from build123d import *

# Parameters (mm, degrees)
SKETCH1_W                = 39.6
SKETCH1_H                = 30
BOSS_EXTRUDE1_DEPTH      = 5
BOSS_EXTRUDE2_DEPTH      = 5.25
BOSS_EXTRUDE2_DEPTH_BACK = 4.75
BOSS_EXTRUDE3_DEPTH      = 5.25
BOSS_EXTRUDE3_DEPTH_BACK = 4.75
SKETCH4_W                = 39.6
SKETCH4_H                = 5
BOSS_EXTRUDE4_DEPTH      = 5.25
SKETCH5_W                = 39.6
SKETCH5_H                = 5
BOSS_EXTRUDE5_DEPTH      = 5.25
SKETCH8_W                = 39.6
SKETCH8_H                = 40.5
BOSS_EXTRUDE6_DEPTH      = 5
SKETCH9_W                = 35.6
SKETCH9_H                = 16.5
CUT_EXTRUDE1_DEPTH       = 2
HOLE1_START              = -5.25
HOLE1_OUTLINE_R          = 2.5
HOLE1_DEPTH              = 40.5
HOLE2_START              = -5.25
HOLE2_OUTLINE_R          = 2.5
HOLE2_DEPTH              = 40.5


# Read off the part's stored shape, not the designer's step: Hole1, Hole2
with BuildPart() as part:
    # Sketch1 → Boss-Extrude1 (new body)
    with BuildSketch(Plane.XY):
        with Locations((19.8, 15)):
            Rectangle(SKETCH1_W, SKETCH1_H)
    extrude(amount=BOSS_EXTRUDE1_DEPTH)

    # Sketch2 → Boss-Extrude2 (add, two sides: drawn at the far end of the back side and taken through both)
    with BuildSketch(Plane.XZ.offset(-BOSS_EXTRUDE2_DEPTH_BACK)):
        Polygon((0, 5), (0, 31.975), (19.798989873, 12.176010127), (39.6, 31.977020254), (39.6, 5), align=None)
    extrude(amount=BOSS_EXTRUDE2_DEPTH + BOSS_EXTRUDE2_DEPTH_BACK)

    # Sketch3 → Boss-Extrude3 (add, two sides: drawn at the far end of the back side and taken through both)
    with BuildSketch(Plane(origin=(0, 30, 0), x_dir=(1, 0, 0), z_dir=(0, 1, 0)).offset(-BOSS_EXTRUDE3_DEPTH_BACK)):
        Polygon((0, -5), (0, -31.975), (19.798989873, -12.176010127), (39.6, -31.977020254), (39.6, -5), align=None)
    extrude(amount=BOSS_EXTRUDE3_DEPTH + BOSS_EXTRUDE3_DEPTH_BACK)

    # Sketch4 → Boss-Extrude4 (add)
    with BuildSketch(Plane(origin=(0, 30, 0), x_dir=(1, 0, 0), z_dir=(0, 1, 0))):
        with Locations((19.8, -2.5)):
            Rectangle(SKETCH4_W, SKETCH4_H)
    extrude(amount=BOSS_EXTRUDE4_DEPTH)

    # Sketch5 → Boss-Extrude5 (add)
    with BuildSketch(Plane.XZ):
        with Locations((19.8, 2.5)):
            Rectangle(SKETCH5_W, SKETCH5_H)
    extrude(amount=BOSS_EXTRUDE5_DEPTH)

    # Sketch8 → Boss-Extrude6 (add)
    with BuildSketch(Plane(origin=(0, 0, 0), x_dir=(-1, 0, 0), z_dir=(0, 0, -1))):
        with Locations((-19.8, 15)):
            Rectangle(SKETCH8_W, SKETCH8_H)
    extrude(amount=BOSS_EXTRUDE6_DEPTH)

    # Sketch9 → Cut-Extrude1 (cut)
    with BuildSketch(Plane.XY.offset(5)):
        with Locations((19.8, 15)):
            Rectangle(SKETCH9_W, SKETCH9_H)
    extrude(amount=-CUT_EXTRUDE1_DEPTH, mode=Mode.SUBTRACT)

    # Hole1 outline → Hole1 (cut)
    with BuildSketch(Plane(origin=(0, 0, 0), x_dir=(1, 0, 0), z_dir=(0, 1, 0)).offset(HOLE1_START)):
        with Locations((7.9, -14.175505063)):
            Circle(HOLE1_OUTLINE_R)
    extrude(amount=HOLE1_DEPTH, mode=Mode.SUBTRACT)

    # Hole2 outline → Hole2 (cut)
    with BuildSketch(Plane(origin=(0, 0, 0), x_dir=(1, 0, 0), z_dir=(0, 1, 0)).offset(HOLE2_START)):
        with Locations((31.7, -14.177525317)):
            Circle(HOLE2_OUTLINE_R)
    extrude(amount=HOLE2_DEPTH, mode=Mode.SUBTRACT)


solid = part.part
Geometry check sheet. Reference: the model listing, model coordinates, mm. A direction names the side the tool comes from. Round coordinates to 2 decimals unless told otherwise and drop trailing zeros. Order: outer loops, then holes, each group sorted by start corner. A loop starts at its lowest first (then second) coordinate and runs counter-clockwise, first axis right, second up. Notation, with made-up numbers: (22, 44.5) -> (61, 44.5) arc R30 cw to (61, 79.5) -> close; hole circle Ø6 at (61, 77.25). An arc over 180 degrees is marked (long way). Use one line per item in the form item = value.
1. Cross-section at B-B, the plane y = 13.5. Enter the section's corners in (x, z), plus the area to 3 significant figures.
Working result:
outline = (0, -5) -> (39.6, -5) -> (39.6, 5) -> (37.6, 5) -> (37.6, 3) -> (2, 3) -> (2, 5) -> (0, 5) -> close
area = 325 mm^2
2. Cross-section at C-C, the plane x = 6.5. Enter the section's corners in (y, z) (3 decimals), plus the area to 3 significant figures.
Working result:
outline = (-5.25, -5) -> (35.25, -5) -> (35.25, 12.104) -> (25.25, 12.104) -> (25.25, 5) -> (23.25, 5) -> (23.25, 3) -> (6.75, 3) -> (6.75, 5) -> (4.75, 5) -> (4.75, 12.104) -> (-5.25, 12.104) -> close; (-5.25, 16.247) -> (4.75, 16.247) -> (4.75, 25.475) -> (-5.25, 25.475) -> close; (25.25, 16.247) -> (35.25, 16.247) -> (35.25, 25.475) -> (25.25, 25.475) -> close
area = 699 mm^2
3. Scan lines: line 1 along Y through (x, z) = (5, 13); line 2 along Z through (x, y) = (25.5, 21); line 3 along X through (y, z) = (28.5, 14) (3 decimals). Record each from-to range of solid material in increasing order. Write a range as from..to.
Working result:
line_1 = -5.25..4.75, 25.25..35.25
line_2 = -5..3
line_3 = 0..5.406, 10.394..17.975, 21.623..29.206, 34.194..39.6
4. Cross-section at D-D, the plane z = 19. Enter the section's corners in (x, y) (3 decimals).
Working result:
outline = (0, -5.25) -> (12.975, -5.25) -> (12.975, 4.75) -> (0, 4.75) -> close; (0, 25.25) -> (12.975, 25.25) -> (12.975, 35.25) -> (0, 35.25) -> close; (26.623, -5.25) -> (39.6, -5.25) -> (39.6, 4.75) -> (26.623, 4.75) -> close; (26.623, 25.25) -> (39.6, 25.25) -> (39.6, 35.25) -> (26.623, 35.25) -> close
5. Go/stop test with flat-tipped pins: pin 1 (6 mm diameter, centred on x = 7.9, z = 14.18, fed in from -Y); pin 2 (6 mm diameter, centred on x = 27.5, y = 23, fed in from +Z); pin 3 (6 mm diameter, centred on x = 11, y = 13, fed in from +Z). Record where each tip stops, or that it passes through.
Working result:
pin_1 = -5.25
pin_2 = 21.86
pin_3 = 3
6. Mould release check, pull along X, two halves, no side actions. Record for faces 1 (the face through (5.92, 30.18, 15.7)), 2 (the face through (20, 6, 5)), 3 (the face through (0, 15, 1)), 4 (the face through (39.6, 15, 1)): pulls with the +X half, pulls with the -X half, needs draft (parallel to the pull), parting line crosses it, or undercut.
Working result:
face_1 = undercut
face_2 = needs draft
face_3 = pulls with the -X half
face_4 = pulls with the +X half
7. Set-up check for faces 5 (the face through (29.561, 30.18, 21.938)), 6 (the face through (29.2, 30.2, 14.1)), 7 (the face through (20, 15, 3)), 8 (the face through (20, 25.25, 12)): record each of +Z, -Z, +X, -X, +Y, -Y from which the full face is reachable in a straight line by a thin tool's end or side.
Working result:
face_5 = +Z, +Y, -Y
face_6 = +Y, -Y
face_7 = +Z
face_8 = +Z, +X, -X
8. Cross-section at A-A, the plane z = 15. Count the separate pieces of the cut face and the enclosed holes in it, plus the area to 3 significant figures.
Working result:
separate_pieces = 8
enclosed_holes = 0
area = 490 mm^2
